Part model, mm, in its own coordinate system. A direction names the side the tool comes from. Coordinates: 2 decimals unless noted, no trailing zeros. Write each loop counter-clockwise with the first axis right and the second up, starting at its lowest first coordinate (ties: lowest second). Pieces come first, ordered by that corner, then holes. Notation, with made-up numbers: (17.5, 5.5) - (52.5, 5.5) arc R27 cw to (52.5, 35.5) - close; hole circle Ø9 at (-4.75, 44.5). An arc over 180 degrees is marked (long way). Use a Markdown table: item, result.
```python
from build123d import *

# Parameters (mm, degrees)
SKETCH1_R                                      = 1.905
BOSS_EXTRUDE2_DEPTH                            = 25.4
CSK_FOR_6_OVAL_HEAD_MACHINE_SCREW1_D           = 3.6576
CSK_FOR_6_OVAL_HEAD_MACHINE_SCREW1_CSINK_D     = 7.0866
CSK_FOR_6_OVAL_HEAD_MACHINE_SCREW1_CSINK_ANGLE = 82


with BuildPart() as part:
    # Sketch1 → Boss-Extrude2 (new body)
    with BuildSketch(Plane(origin=(0, 0, 0), x_dir=(1, 0, 0), z_dir=(0, 1, 0))):
        Polygon((0, 0), (-28.124290221, 0), (-28.124290221, 12.7), (0, 12.7), (0, 19.05), (0, 69.85), (-11.938801262, 69.85), (-11.938801262, 19.05), (-38.1, 19.05), (-38.1, 7.031072555), (-38.1, -6.35), (0, -6.35), align=None)
        with Locations(Location((-5.969400631, 57.15, 0), (0, 0, 270))):
            Circle(SKETCH1_R, mode=Mode.SUBTRACT)
    extrude(amount=BOSS_EXTRUDE2_DEPTH)

    # CSK for #6 Oval Head Machine Screw1 (through all)
    with Locations(Plane(origin=(0, 0, -19.05), x_dir=(-1, 0, 0), z_dir=(0, 0, -1))):
        with Locations((18.479100946, 12.7)):
            CounterSinkHole(CSK_FOR_6_OVAL_HEAD_MACHINE_SCREW1_D / 2, CSK_FOR_6_OVAL_HEAD_MACHINE_SCREW1_CSINK_D / 2, counter_sink_angle=CSK_FOR_6_OVAL_HEAD_MACHINE_SCREW1_CSINK_ANGLE)


solid = part.part
```
Item 1: Two-plate mould, pull along X, no slides. Class faces 1 (the face through (-25, 13, -19.05)), 2 (the face through (-20, 11.5, -17.2)), 3 (the face through (-38.1, 13, -7)): pulls with the +X half, pulls with the -X half, needs draft (parallel to the pull), parting line crosses it, or undercut.
From the geometry:
| item | result |
|---|---|
| face 1 | needs draft |
| face 2 | undercut |
| face 3 | pulls with the -X half |
Item 2: Drop flat-ended pins along their axis: P1, Ø1.5, axis at x = -29, y = 21, coming from the -Z side; P2, Ø4, axis at y = 17, z = -8, coming from the +X side; P3, Ø3.5, axis at x = -5.97, z = -57.15, coming from the -Y side; P4, Ø4, axis at x = -18.48, y = 12.7, coming from the -Z side. Give the stop position or say it passes through.
From the geometry:
| item | result |
|---|---|
| P1 | z = -19.05 |
| P2 | x = -28.12 |
| P3 | through |
| P4 | z = -17.28 |
Item 3: Band-saw the part on A-A, the plane y = 12.7. Give the cut face in (x, z) (3 decimals).
From the geometry:
| item | result |
|---|---|
| outline | (-38.1, -19.05) - (-22.022, -19.05) - (-20.308, -17.078) - (-20.308, -12.7) - (-28.124, -12.7) - (-28.124, 0) - (-20.308, 0) - (-20.308, 6.35) - (-38.1, 6.35) - close; (-16.65, -17.078) - (-14.936, -19.05) - (-11.939, -19.05) - (-11.939, -69.85) - (0, -69.85) - (0, -12.7) - (-16.65, -12.7) - close; (-16.65, 0) - (0, 0) - (0, 6.35) - (-16.65, 6.35) - close; hole circle Ø3.81 at (-5.969, -57.15) |
Item 4: Band-saw the part on D-D, the plane x = -18. Count the separate pieces of the cut face and the enclosed holes in it, then the cut area to 3 significant figures.
From the geometry:
| item | result |
|---|---|
| separate pieces | 4 |
| enclosed holes | 0 |
| area | 274 mm^2 |
Item 5: Which spindle directions (+Z, -Z, +X, -X, +Y, -Y) get a long thin tool onto all of the face, cutting with end or side? Do faces 4 (the face through (-14, 13, 0)), 5 (the face through (-5.4, 12.52, -55.33)), 6 (the face through (-11.939, 13, -45)). Say none if no direction does.
From the geometry:
| item | result |
|---|---|
| face 4 | +X, +Y, -Y |
| face 5 | +Y, -Y |
| face 6 | -Z, -X, +Y, -Y |
Item 6: Band-saw the part on B-B, the plane z = -57.15. Give the cut face in (x, y).
From the geometry:
| item | result |
|---|---|
| outline | (-11.94, 0) - (-7.87, 0) - (-7.87, 25.4) - (-11.94, 25.4) - close; (-4.06, 0) - (0, 0) - (0, 25.4) - (-4.06, 25.4) - close |
Item 7: Band-saw the part on C-C, the plane y = 5. Give the cut face in (x, z) (3 decimals).
From the geometry:
| item | result |
|---|---|
| outline | (-38.1, -19.05) - (-11.939, -19.05) - (-11.939, -69.85) - (0, -69.85) - (0, -12.7) - (-28.124, -12.7) - (-28.124, 0) - (0, 0) - (0, 6.35) - (-38.1, 6.35) - close; hole circle Ø3.81 at (-5.969, -57.15) |
Item 8: Drill centre lines: probe 1 along X at (y, z) = (12.7, -13.7); probe 2 along Z at (x, y) = (-13, 1). Where is each one in solid material? Low to high.
From the geometry:
| item | result |
|---|---|
| probe 1 | -38.1 to -20.31, -16.65 to 0 |
| probe 2 | -19.05 to -12.7, 0 to 6.35 |
